from build123d import *

# Parameters (mm, degrees)
F0_W      = 777
F0_H      = 682
F1_DEPTH  = 12
F2_W      = 777
F2_H      = 6
F3_DEPTH  = 6
F4_W      = 637
F4_H      = 170
F5_DEPTH  = 12
F6_W      = 777
F6_H      = 6
F7_DEPTH  = 6
F8_W      = 6
F8_H      = 676
F9_DEPTH  = 6
F10_W     = 6
F10_H     = 676
F11_DEPTH = 6
F12_W     = 765
F12_H     = 6
F13_DEPTH = 6


with BuildPart() as f1:
    # F0 (on Front) → F1 (new body)
    with BuildSketch(Plane.XZ):
        Rectangle(F0_W, F0_H)
    extrude(amount=F1_DEPTH)

    # F2 (on face) → F3 (cut)
    with BuildSketch(Plane.XZ.offset(12)):
        with Locations((0, 108)):
            Rectangle(F2_W, F2_H)
    extrude(amount=-F3_DEPTH, mode=Mode.SUBTRACT)

    # F4 (on face) → F5 (cut, through all)
    with BuildSketch(Plane.XZ.offset(12)):
        with Locations((-10, 206)):
            Rectangle(F4_W, F4_H)
    extrude(amount=-F5_DEPTH, mode=Mode.SUBTRACT)

    # F6 (on face) → F7 (cut)
    with BuildSketch(Plane.XZ.offset(12)):
        with Locations((0, 338)):
            Rectangle(F6_W, F6_H)
    extrude(amount=-F7_DEPTH, mode=Mode.SUBTRACT)

    # F8 (on face) → F9 (cut)
    with BuildSketch(Plane.XZ.offset(12)):
        with Locations((-385.5, -3)):
            Rectangle(F8_W, F8_H)
    extrude(amount=-F9_DEPTH, mode=Mode.SUBTRACT)

    # F10 (on face) → F11 (cut)
    with BuildSketch(Plane.XZ.offset(12)):
        with Locations((385.5, -3)):
            Rectangle(F10_W, F10_H)
    extrude(amount=-F11_DEPTH, mode=Mode.SUBTRACT)

    # F12 (on face) → F13 (cut)
    with BuildSketch(Plane.XZ.offset(12)):
        with Locations((0, -338)):
            Rectangle(F12_W, F12_H)
    extrude(amount=-F13_DEPTH, mode=Mode.SUBTRACT)


solid = f1.part
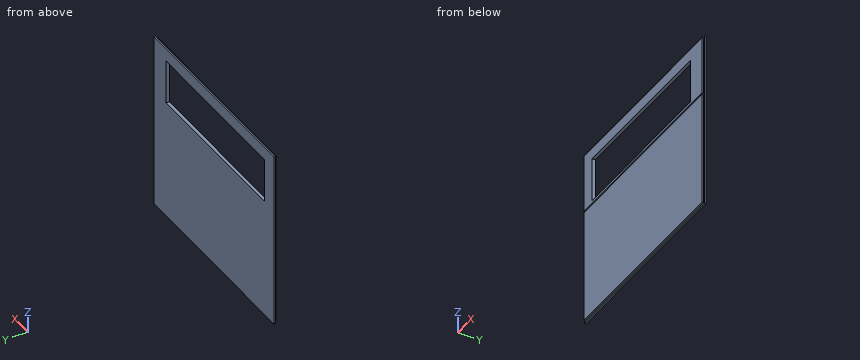
Input: part model. Units: mm. Frame: model coordinates. Give positions to 0.01 mm unless a question says otherwise; leave off trailing zeros. Order: outer loops, then holes, each group sorted by start corner. A loop starts at its lowest first (then second) coordinate and runs counter-clockwise, first axis right, second up.
Q1. Section A-A on y = -9.75. Output: boundary loops of the cut face in (x, z).
Checked values:
outline: (-382.5, -335) - (382.5, -335) - (382.5, 105) - (-382.5, 105) - close; (-382.5, 111) - (382.5, 111) - (382.5, 335) - (-382.5, 335) - close; hole (-328.5, 121) - (308.5, 121) - (308.5, 291) - (-328.5, 291) - close
Q2. Ray query, probe 1 along Z at (x, y) = (3, -9.75); probe 2 along Z at (x, y) = (-297, -2.25); probe 3 along X at (y, z) = (-4.5, 198). Return the intervals inside material, ascending.
Checked values:
probe 1: z = -335 to 105, 111 to 121, 291 to 335
probe 2: z = -341 to 121, 291 to 341
probe 3: x = -388.5 to -328.5, 308.5 to 388.5
Q3. Contact query for flat-ended pins moving along their axis: pin 1 Ø1.8 at (y, z) = (-8.5, 252.5) entering from +X; pin 2 Ø3.5 at (x, y) = (-62.5, -8.5) entering from +Z; pin 3 Ø3 at (x, y) = (-121.5, -8) entering from -Z. Output: stop coordinate, or through.
Checked values:
pin 1: stops at x = 382.5
pin 2: stops at z = 335
pin 3: stops at z = -335
Q4. Section C-C on z = 216.5. Output: boundary loops of the cut face in (x, y), and give its area (3 significant figures).
Checked values:
outline: (-388.5, -6) - (-382.5, -6) - (-382.5, -12) - (-328.5, -12) - (-328.5, 0) - (-388.5, 0) - close; (308.5, -12) - (382.5, -12) - (382.5, -6) - (388.5, -6) - (388.5, 0) - (308.5, 0) - close
area: 1,610 mm2
Q5. Section B-B on x = 65.5. Output: boundary loops of the cut face in (y, z), and give its area (3 significant figures).
Checked values:
outline: (-12, -335) - (-6, -335) - (-6, -341) - (0, -341) - (0, 121) - (-12, 121) - (-12, 111) - (-6, 111) - (-6, 105) - (-12, 105) - close; (-12, 291) - (0, 291) - (0, 341) - (-6, 341) - (-6, 335) - (-12, 335) - close
area: 6,040 mm2
